Here's how the part is built. I have some questions about the finished solid (model axes, mm). Coordinates: 2 decimals unless noted, no trailing zeros. Loops run counter-clockwise (first coordinate to the right, second up) from the corner with the lowest first, then second, coordinate; pieces in that order, holes last. Notation, with made-up numbers: (-8, 68.25) - (29, 68.25) arc R14 cw to (29, 80.25) - close; hole circle Ø10 at (47.5, -6). An arc over 180 degrees is marked (long way). Use a Markdown table: item, result.
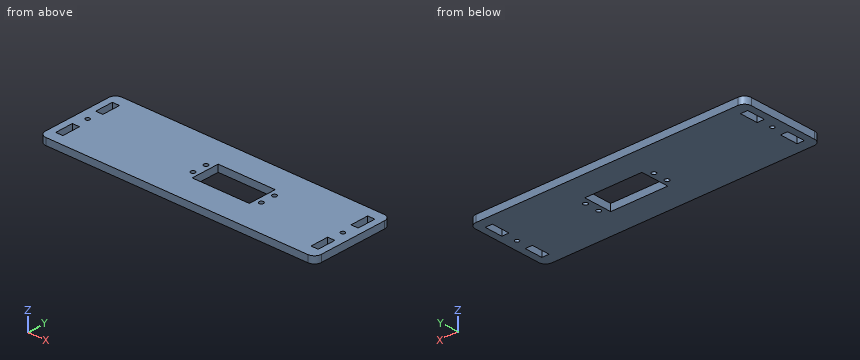
```python
from build123d import *

# Parameters (mm, degrees)
SKETCH1_R           = 1.6
SKETCH1_R_2         = 1.5
SKETCH1_W           = 5.2
SKETCH1_H           = 13.2
SKETCH1_W_2         = 41.4
SKETCH1_H_2         = 20.5
BOSS_EXTRUDE1_DEPTH = 5


with BuildPart() as part:
    # Sketch1 → Boss-Extrude1 (new body)
    with BuildSketch(Plane.XY):
        with BuildLine():
            Line((-36.027647281, 22.573731276), (153.972352719, 22.573731276))
            ThreePointArc((153.972352719, 22.573731276), (157.507886625, 21.109265182), (158.972352719, 17.573731276))
            Line((158.972352719, 17.573731276), (158.972352719, -32.426268724))
            ThreePointArc((158.972352719, -32.426268724), (157.507886625, -35.96180263), (153.972352719, -37.426268724))
            Line((153.972352719, -37.426268724), (-36.027647281, -37.426268724))
            ThreePointArc((-36.027647281, -37.426268724), (-39.563181187, -35.96180263), (-41.027647281, -32.426268724))
            Line((-41.027647281, -32.426268724), (-41.027647281, 17.573731276))
            ThreePointArc((-41.027647281, 17.573731276), (-39.563181187, 21.109265182), (-36.027647281, 22.573731276))
        make_face()
        with Locations((47.372352719, -1.826397645)):
            Circle(SKETCH1_R, mode=Mode.SUBTRACT)
        with Locations((47.372352719, -12.226397645)):
            Circle(SKETCH1_R, mode=Mode.SUBTRACT)
        with Locations((96.972352719, -12.226397645)):
            Circle(SKETCH1_R, mode=Mode.SUBTRACT)
        with Locations((96.972352719, -1.826397645)):
            Circle(SKETCH1_R, mode=Mode.SUBTRACT)
        with Locations((151.369386748, -7.026268724)):
            Circle(SKETCH1_R_2, mode=Mode.SUBTRACT)
        with Locations(Location((-33.42468131, -7.426268724, 0), (0, 0, 180))):
            Circle(SKETCH1_R_2, mode=Mode.SUBTRACT)
        with Locations((-33.42468131, 8.373731276)):
            Rectangle(SKETCH1_W, SKETCH1_H, mode=Mode.SUBTRACT)
        with Locations((151.369386748, -22.826268724)):
            Rectangle(SKETCH1_W, SKETCH1_H, mode=Mode.SUBTRACT)
        with Locations((151.369386748, 8.773731276)):
            Rectangle(SKETCH1_W, SKETCH1_H, mode=Mode.SUBTRACT)
        with Locations((72.172352719, -7.026268724)):
            Rectangle(SKETCH1_W_2, SKETCH1_H_2, mode=Mode.SUBTRACT)
        with Locations((-33.42468131, -23.226268724)):
            Rectangle(SKETCH1_W, SKETCH1_H, mode=Mode.SUBTRACT)
    extrude(amount=BOSS_EXTRUDE1_DEPTH)


solid = part.part
```
Q1. I want a section at A-A, the plane x = 73.5. Write out the boundary of the cut face in (y, z), then the cut area to 4 significant figures.
Check values:
| item | result |
|---|---|
| outline | (-37.43, 0) - (-17.28, 0) - (-17.28, 5) - (-37.43, 5) - close; (3.22, 0) - (22.57, 0) - (22.57, 5) - (3.22, 5) - close |
| area | 197.5 mm^2 |
Q2. Please list where these lines run through material, in increasing order: L1, parallel to X at y = 12, z = 4.5; L2, parallel to X at y = -12.5, z = 4.45; L3, parallel to X at y = -16, z = 3.5. Write a range as from..to.
Check values:
| item | result |
|---|---|
| L1 | -41.03..-36.02, -30.82..148.77, 153.97..158.97 |
| L2 | -41.03..45.8, 48.95..51.47, 92.87..95.4, 98.55..158.97 |
| L3 | -41.03..51.47, 92.87..158.97 |
Q3. Will these pins go through, and if not, where does the flat tip stop? P1, Ø1.9, axis at x = 96.97, y = -12.23, coming from the -Z side; P2, Ø5, axis at x = 96.97, y = -1.83, coming from the -Z side.
Check values:
| item | result |
|---|---|
| P1 | through |
| P2 | z = 0 |
Q4. I want a section at C-C, the plane z = 1.55. Give the number of separate pieces and of enclosed holes in the cut face, then the cut area to 3 significant figures.
Check values:
| item | result |
|---|---|
| separate pieces | 1 |
| enclosed holes | 11 |
| area | 10,800 mm^2 |
Q5. I want a section at B-B, the plane y = 6. Write out the boundary of the cut face in (x, z).
Check values:
| item | result |
|---|---|
| outline | (-41.03, 0) - (-36.02, 0) - (-36.02, 5) - (-41.03, 5) - close; (-30.82, 0) - (148.77, 0) - (148.77, 5) - (-30.82, 5) - close; (153.97, 0) - (158.97, 0) - (158.97, 5) - (153.97, 5) - close |
